Work out the finished part from the listing and answer in its coordinate system (mm). Give positions to 0.01 mm unless a question says otherwise; leave off trailing zeros. Order: outer loops, then holes, each group sorted by start corner. A loop starts at its lowest first (then second) coordinate and runs counter-clockwise, first axis right, second up. Notation, with made-up numbers: (13, -16) -> (66, -16) arc R19 ccw to (66, 12) -> close; hole circle Ø9 at (59, 27.25). An arc over 180 degrees is marked (long way). Answer as CSV lines item,"result". Start each with the question number.
1. Find the intervals of material crossed by L1, parallel to Y at x = 133.2, z = 0; L2, parallel to Z at x = 134.4, y = -21.1; L3, parallel to Y at x = 132.1, z = 20.5, in increasing order.
2. A cutting plane is placed at B-B (y = 0). Give the vertices of the cut face in (x, z).
3. A cutting plane is placed at C-C (z = 19.5). Give the vertices of the cut face in (x, y).
4. Flat-ended cylindrical pins translate along their axes: pin 1 (12 mm diameter, centred on y = -35.5, z = -36, fed in from -X); pin 2 (2 mm diameter, centred on x = 133, y = -31, fed in from -Z); pin 3 (1 mm diameter, centred on x = 134.5, y = -11, fed in from +Z); pin 4 (1 mm diameter, centred on x = 133, z = -34.5, fed in from -Y). Find the tip coordinate at first contact, or state that the pin passes through.
5. For a pull along Z with two mould halves and no side action, classify faces 1 (the cylindrical face through (133.73, -45.61, -5.99)), 2 (the cylindrical face through (133.67, 43.59, -0.89)), 3 (the flat face through (131.7, 20, -20)) as released by +Z, released by -Z, zero draft, split by the parting line, or undercut.
6. A cutting plane is placed at D-D (x = 132.9). Give the vertices of the cut face in (y, z).
7. A cutting plane is placed at A-A (z = 0). Give the vertices of the cut face in (x, y), then the cut area to 3 significant figures.
from build123d import *

# Parameters (mm, degrees)
AXIAL_PROFILE_MM_W     = 4
AXIAL_PROFILE_MM_H     = 19
AXIAL_HOLES_DEPTH      = 151.487507787
AXIAL_HOLES_DEPTH_BACK = 151.487507787
SKETCH2_R              = 1.65


with BuildPart() as part:
    # Axial profile (mm) → Full revolution (revolve)
    with BuildSketch(Plane.XY, mode=Mode.PRIVATE) as full_revolution_sk:
        with Locations((133.7, 36.5)):
            Rectangle(AXIAL_PROFILE_MM_W, AXIAL_PROFILE_MM_H)
    revolve(full_revolution_sk.sketch.rotate(Axis((-110, 0, 0), (1, 0, 0)), 90), axis=Axis((-110, 0, 0), (1, 0, 0)))

    # Sketch2 → Axial holes (cut, two sides: drawn at the far end of the back side and taken through both)
    with BuildSketch(Plane(origin=(0, 0, 0), x_dir=(0, 0, -1), z_dir=(1, 0, 0)).offset(-AXIAL_HOLES_DEPTH_BACK)):
        with Locations((0, 42.2)):
            Circle(SKETCH2_R)
        with Locations((-36.54627204, -21.1)):
            Circle(SKETCH2_R)
        with Locations((36.54627204, -21.1)):
            Circle(SKETCH2_R)
    extrude(amount=AXIAL_HOLES_DEPTH + AXIAL_HOLES_DEPTH_BACK, mode=Mode.SUBTRACT)


solid = part.part
Answer sheet:
1,L1,"y = -46 to -27, 27 to 40.55, 43.85 to 46"
1,L2,"z = -40.88 to -38.2, -34.9 to -16.85, 16.85 to 34.9, 38.2 to 40.88"
1,L3,"y = -41.18 to -17.57, 17.57 to 41.18"
2,outline,"(131.7, -46) -> (135.7, -46) -> (135.7, -27) -> (131.7, -27) -> close; (131.7, 27) -> (135.7, 27) -> (135.7, 46) -> (131.7, 46) -> close"
3,outline,"(131.7, -41.66) -> (135.7, -41.66) -> (135.7, -18.67) -> (131.7, -18.67) -> close; (131.7, 18.67) -> (135.7, 18.67) -> (135.7, 41.66) -> (131.7, 41.66) -> close"
4,pin 1,"stops at x = 131.7"
4,pin 2,"stops at z = -34.87"
4,pin 3,"stops at z = 44.79"
4,pin 4,"stops at y = -30.98"
5,face 1,"split by the parting line"
5,face 2,"undercut"
5,face 3,"zero draft"
6,outline,"circle Ø92 at (0, 0); hole circle Ø54 at (0, 0); hole circle Ø3.3 at (-21.1, -36.55); hole circle Ø3.3 at (-21.1, 36.55); hole circle Ø3.3 at (42.2, 0)"
7,outline,"(131.7, -46) -> (135.7, -46) -> (135.7, -27) -> (131.7, -27) -> close; (131.7, 27) -> (135.7, 27) -> (135.7, 40.55) -> (131.7, 40.55) -> close; (131.7, 43.85) -> (135.7, 43.85) -> (135.7, 46) -> (131.7, 46) -> close"
7,area,"139 mm^2"
